Check sheet for the modelled part. Datum: model origin and axes. Units: mm. Face numbers are marked on the shaded views. A direction names the side the tool comes from. Coordinates: 2 decimals unless noted, no trailing zeros. Write each loop counter-clockwise with the first axis right and the second up, starting at its lowest first coordinate (ties: lowest second). Pieces come first, ordered by that corner, then holes. Notation, with made-up numbers: (-37, 6) - (5, 6) arc R29 cw to (5, 27) - close; hole circle Ø6 at (25, 21). An arc over 180 degrees is marked (long way). Write each question's results on one line, items separated by ' | '.
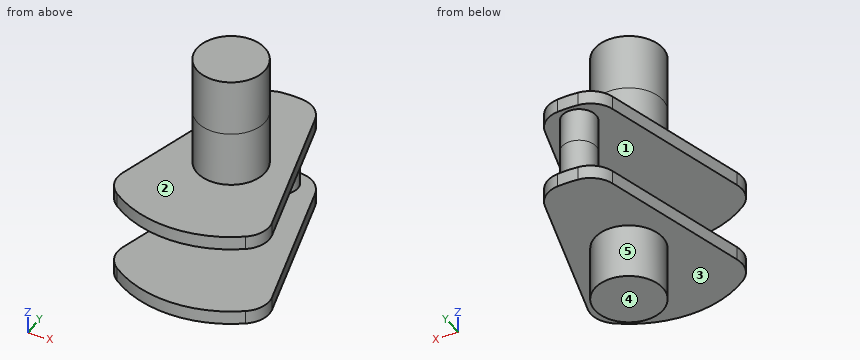
from build123d import *

# Parameters (mm, degrees)
BOSS_EXTRUDE1_DEPTH = 0.8
SKETCH3_R           = 1
BOSS_EXTRUDE2_DEPTH = 2
SKETCH4_R           = 2
BOSS_EXTRUDE3_DEPTH = 3.26
SKETCH5_R           = 2
BOSS_EXTRUDE4_DEPTH = 3.34
SKETCH6_W           = 0.1
SKETCH6_H           = 0.5
CUT_EXTRUDE1_DEPTH  = 0.1


with BuildPart() as part:
    # Sketch2 → Boss-Extrude1 (new body)
    with BuildSketch(Plane.XY):
        with BuildLine():
            Line((-2.002843202, 5.298630925), (-4.411867861, -3.552786589))
            ThreePointArc((-4.411867861, -3.552786589), (-4.376483825, -4.506396112), (-3.804522508, -5.270256966))
            ThreePointArc((-3.804522508, -5.270256966), (0, -6.5), (3.804522508, -5.270256966))
            ThreePointArc((3.804522508, -5.270256966), (4.376483825, -4.506396112), (4.411867861, -3.552786589))
            Line((4.411867861, -3.552786589), (2.002843202, 5.298630925))
            ThreePointArc((2.002843202, 5.298630925), (1.489063424, 6.102778606), (0.608877551, 6.471419329))
            ThreePointArc((0.608877551, 6.471419329), (0, 6.5), (-0.608877551, 6.471419329))
            ThreePointArc((-0.608877551, 6.471419329), (-1.489063424, 6.102778606), (-2.002843202, 5.298630925))
        make_face()
    extrude(amount=BOSS_EXTRUDE1_DEPTH)

    # Sketch3 → Boss-Extrude2 (add)
    with BuildSketch(Plane.XY.offset(0.8)):
        with Locations((0, 5.26)):
            Circle(SKETCH3_R)
    extrude(amount=BOSS_EXTRUDE2_DEPTH)

    # Sketch4 → Boss-Extrude3 (add)
    with BuildSketch(Plane(origin=(0, 0, 0), x_dir=(-1, 0, 0), z_dir=(0, 0, -1))):
        Circle(SKETCH4_R)
    extrude(amount=BOSS_EXTRUDE3_DEPTH)

    # Mirror1: part across plane


with BuildPart() as part_1:
    add(part.part)
    add(part.part.mirror(Plane(origin=(0, 5.26, 2.8), x_dir=(1, 0, 0), z_dir=(0, 0, 1))))

    # Sketch5 → Boss-Extrude4 (add)
    with BuildSketch(Plane.XY.offset(8.86)):
        Circle(SKETCH5_R)
    extrude(amount=BOSS_EXTRUDE4_DEPTH)

    # Sketch6 → Cut-Extrude1 (cut)
    with BuildSketch(Plane.XY.offset(5.6)):
        with Locations((0.05, 2.280573289)):
            Rectangle(SKETCH6_W, SKETCH6_H)
    extrude(amount=-CUT_EXTRUDE1_DEPTH, mode=Mode.SUBTRACT)


solid = part_1.part
1. Sectioned sample at D-D (y = -2.5). Record the cut outline in (x, z).
Values follow:
outline: (-4.13, 0) - (4.13, 0) - (4.13, 0.8) - (-4.13, 0.8) - close; (-4.13, 4.8) - (4.13, 4.8) - (4.13, 5.6) - (-4.13, 5.6) - close
2. Sectioned sample at A-A (y = 0.5). Record the cut outline in (x, z), then the cut area to 3 significant figures.
Values follow:
outline: (-3.31, 0) - (-1.94, 0) - (-1.94, -3.26) - (1.94, -3.26) - (1.94, 0) - (3.31, 0) - (3.31, 0.8) - (-3.31, 0.8) - close; (-3.31, 4.8) - (3.31, 4.8) - (3.31, 5.6) - (1.94, 5.6) - (1.94, 12.2) - (-1.94, 12.2) - (-1.94, 5.6) - (-3.31, 5.6) - close | area: 48.8 mm^2
3. Go/stop test with flat-tipped pins: pin 1 (2.5 mm diameter, centred on x = 1.5, y = 2.5, fed in from -Z); pin 2 (1 mm diameter, centred on x = 0.5, y = 2.5, fed in from -Z); pin 3 (2 mm diameter, centred on x = 0.5, z = 3.5, fed in from -Y); pin 4 (1 mm diameter, centred on y = 3.5, z = 0, fed in from -X). Record where each tip stops, or that it passes through.
Values follow:
pin 1: stops at z = -3.26 | pin 2: stops at z = 0 | pin 3: stops at y = 4.26 | pin 4: stops at x = -2.63
4. Material ranges on L1, parallel to Z at x = -2, y = -4.25; L2, parallel to Z at x = -1.25, y = 1; L3, parallel to Z at x = 0.25, y = 5, recorded low to high. Write a range as [from, to].
Values follow:
L1: z = [0, 0.8], [4.8, 5.6] | L2: z = [-3.26, 0.8], [4.8, 12.2] | L3: z = [0, 5.6]
5. Sectioned sample at B-B (x = 3.5). Record the cut outline in (y, z).
Values follow:
outline: (-5.48, 0) - (-0.2, 0) - (-0.2, 0.8) - (-5.48, 0.8) - close; (-5.48, 4.8) - (-0.2, 4.8) - (-0.2, 5.6) - (-5.48, 5.6) - close
6. Access from +Z, -Z, +X, -X, +Y, -Y to the whole of each face (thin tool, end or side, straight path). Record for the marked faces 4 and 5.
Values follow:
face 4: -Z, +X, -X, +Y, -Y | face 5: -Z
7. Draft check along Z on the marked faces 1, 2 and 3. Enter one of: pulls with the +Z half, pulls with the -Z half, needs draft (parallel to the pull), parting line crosses it, or undercut.
Values follow:
face 1: undercut | face 2: pulls with the +Z half | face 3: pulls with the -Z half
8. Sectioned sample at C-C (z = 7.25). Record the cut outline in (x, y).
Values follow:
outline: circle Ø4 at (0, 0)
